from build123d import *

# Parameters (mm, degrees)
F0_W     = 50
F0_H     = 50
F1_DEPTH = 2
F2_R     = 1.5
F3_DEPTH = 2.001
F4_W     = 25
F4_H     = 10
F5_DEPTH = 6


with BuildPart() as f1:
    # F0 (on Top) → F1 (new body)
    with BuildSketch(Plane.XY):
        Rectangle(F0_W, F0_H)
    extrude(amount=F1_DEPTH)

    # F2 (on Top) → F3 (cut, through all)
    with BuildSketch(Plane.XY):
        with Locations((-22, 22)):
            Circle(F2_R)
        with Locations((-22, -22)):
            Circle(F2_R)
        with Locations((22, -22)):
            Circle(F2_R)
        with Locations((22, 22)):
            Circle(F2_R)
    extrude(amount=F3_DEPTH, mode=Mode.SUBTRACT)

    # F4 (on face) → F5 (join)
    with BuildSketch(Plane.XY.offset(2)):
        Rectangle(F4_W, F4_H)
    extrude(amount=F5_DEPTH)


solid = f1.part
Here's how the part is built. I have some questions about the finished solid (model axes, mm). A direction names the side the tool comes from. Round coordinates to 2 decimals unless told otherwise and drop trailing zeros. Loops run counter-clockwise (first coordinate to the right, second up) from the corner with the lowest first, then second, coordinate; pieces in that order, holes last. Notation, with made-up numbers: (77, 42) - (109, 42) arc R15 ccw to (109, 49) - close; hole circle Ø11 at (72.25, -18.5). An arc over 180 degrees is marked (long way). One line per question, with ' | ' between items. Start each with the question number.
Q1. Will these pins go through, and if not, where does the flat tip stop? pin 1 (3 mm diameter, centred on x = -5.5, z = 5, fed in from -Y); pin 2 (4 mm diameter, centred on x = 22, y = 22, fed in from +Z).
Q2. I want a section at C-C (y = 1). Write out the boundary of the cut face in (x, z).
Q3. We'd pull the mould along X, two halves only. Please class faces 1 (the flat face through (0, -5, 5)), 2 (the cylindrical face through (-23.11, 23.01, 0.99)), 3 (the flat face through (25, 0, 1)): +X half, -X half, draft (parallel to the pull), parting line (faces both ways), or undercut.
Q4. Please list where these lines run through material, in increasing order: line 1 (Y direction, x = -22, z = 1.5); line 2 (Y direction, x = 21, z = 1). Write a range as [from, to].
Q5. I want a section at D-D (x = -6.5). Write out the boundary of the cut face in (y, z), then the cut area to 3 significant figures.
Q6. I want a section at A-A (x = -22). Write out the boundary of the cut face in (y, z), then the cut area to 3 significant figures.
Q7. For faces 4 (the flat face through (-12.5, 0, 5)), 5 (the flat face through (0, 5, 5)), 6 (the flat face through (12.5, 0, 5)), 7 (the flat face through (0, 25, 1)), which set-ups out of +Z, -Z, +X, -X, +Y, -Y let a thin tool reach every point of the face, with its end or its side?
Response values:
1) pin 1: stops at y = -5 | pin 2: stops at z = 2
2) outline: (-25, 0) - (25, 0) - (25, 2) - (12.5, 2) - (12.5, 8) - (-12.5, 8) - (-12.5, 2) - (-25, 2) - close
3) face 1: draft | face 2: undercut | face 3: +X half
4) line 1: y = [-25, -23.5], [-20.5, 20.5], [23.5, 25] | line 2: y = [-25, -23.12], [-20.88, 20.88], [23.12, 25]
5) outline: (-25, 0) - (25, 0) - (25, 2) - (5, 2) - (5, 8) - (-5, 8) - (-5, 2) - (-25, 2) - close | area: 160 mm²
6) outline: (-25, 0) - (-23.5, 0) - (-23.5, 2) - (-25, 2) - close; (-20.5, 0) - (20.5, 0) - (20.5, 2) - (-20.5, 2) - close; (23.5, 0) - (25, 0) - (25, 2) - (23.5, 2) - close | area: 88.0 mm²
7) face 4: +Z, -X, +Y, -Y | face 5: +Z, +X, -X, +Y | face 6: +Z, +X, +Y, -Y | face 7: +Z, -Z, +X, -X, +Y
